from build123d import *

# Parameters (mm, degrees)
ESBO_O1_W                = 45
ESBO_O1_H                = 50
RESSALTO_EXTRUS_O1_DEPTH = 10
CORTE_EXTRUS_O1_DEPTH    = 7
CORTE_EXTRUS_O2_DEPTH    = 5.5
CHANFRO1_SIZE            = 5.5
ESBO_O4_R                = 1.65
RESSALTO_EXTRUS_O2_DEPTH = 3
CORTE_EXTRUS_O3_DEPTH    = 43.793106922


with BuildPart() as part:
    # Esboço1 → Ressalto-extrusão1 (new body)
    with BuildSketch(Plane.XY):
        Rectangle(ESBO_O1_W, ESBO_O1_H)
    extrude(amount=RESSALTO_EXTRUS_O1_DEPTH)

    # Esboço2 → Corte-extrusão1 (cut)
    with BuildSketch(Plane.XY.offset(10)):
        Polygon((-15, -5), (0, -12), (15, -5), (15, 25), (-15, 25), align=None)
    extrude(amount=-CORTE_EXTRUS_O1_DEPTH, mode=Mode.SUBTRACT)

    # Esboço3 → Corte-extrusão2 (cut)
    with BuildSketch(Plane.XY.offset(3)):
        Polygon((-15, -5), (-15, -12), (0, -19), (15, -12), (15, -5), align=None)
    extrude(amount=CORTE_EXTRUS_O2_DEPTH, mode=Mode.SUBTRACT)

    # Chanfro1
    chanfro1_edges = [part.edges().sort_by_distance(p)[0] for p in [
        (-7.5, -15.5, 8.5),
        (7.5, -15.5, 8.5),
    ]]
    chamfer(chanfro1_edges, length=CHANFRO1_SIZE - 0.0001)  # a hair under: the kernel refuses the full size

    # Esboço4 → Ressalto-extrusão2 (add)
    with BuildSketch(Plane(origin=(0, 0, 0), x_dir=(-1, 0, 0), z_dir=(0, 0, -1))):
        with BuildLine():
            Line((4.245283019, 32.641509434), (9, 25))
            Line((9, 25), (-9, 25))
            Line((-9, 25), (-4.245283019, 32.641509434))
            ThreePointArc((-4.245283019, 32.641509434), (0, 35), (4.245283019, 32.641509434))
        make_face()
        with Locations((0, 30)):
            Circle(ESBO_O4_R, mode=Mode.SUBTRACT)
    extrude(amount=-RESSALTO_EXTRUS_O2_DEPTH)

    # Esboço5 → Corte-extrusão3 (cut, through all)
    with BuildSketch(Plane.XY.offset(10)):
        Polygon((-22.5, -11.431767214), (0, -21.931767214), (22.5, -11.431767214), (22.5, -32.501990612), (-22.5, -32.501990612), align=None)
    extrude(amount=-CORTE_EXTRUS_O3_DEPTH, mode=Mode.SUBTRACT)


solid = part.part
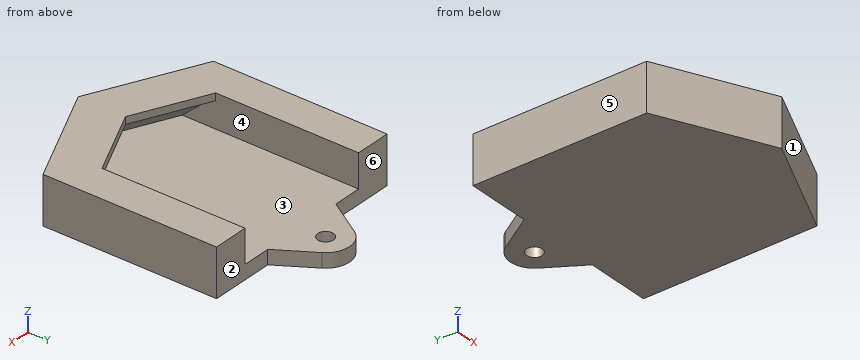
Here's how the part is built. I have some questions about the finished solid (model axes, mm). Face numbers are marked on the shaded views. A direction names the side the tool comes from. Give positions to 0.01 mm unless a question says otherwise; leave off trailing zeros. Loops run counter-clockwise (first coordinate to the right, second up) from the corner with the lowest first, then second, coordinate; pieces in that order, holes last. Notation, with made-up numbers: (29, 88.5) -> (75, 88.5) arc R35 cw to (75, 121.5) -> close; hole circle Ø6 at (0.25, -23.75). An arc over 180 degrees is marked (long way). Answer as a JSON object with one key per item and string values. Group by question number.
Item 1: Imagine slicing it at C-C on y = 30. Write out the boundary of the cut face in (x, z), then the cut area to 3 significant figures.
Item 2: Will these pins go through, and if not, where does the flat tip stop? pin 1 (6.5 mm diameter, centred on x = -1.5, y = -7.5, fed in from -Z); pin 2 (15 mm diameter, centred on x = 6.5, y = 17, fed in from +Z); pin 3 (4 mm diameter, centred on x = -2.5, z = 7.5, fed in from +Y); pin 4 (1.5 mm diameter, centred on x = 4, z = 5, fed in from -Y).
Item 3: Imagine slicing it at A-A on z = 1. Write out the boundary of the cut face in (x, y).
Item 4: On a 3-axis mill with a long thin cutter (end or side, diameter ignored), from which of +Z, -Z, +X, -X, +Y, -Y can I reach the whole of each face in a straight line? I mean the marked faces 4, 5 and 6. Say none if no direction works.
Item 5: Thinking about a two-plate mould opening in Y: for the marked faces 1, 2 and 3, which applies, pulls with the +Y half, pulls with the -Y half, needs draft (parallel to the pull), parting line crosses it, or undercut?
Item 6: I need wall thicknesses on L1, parallel to X at y = 17.5, z = 6.5; L2, parallel to Y at x = 0, z = 1.65; L3, parallel to Z at x = -2, y = 6.5. Which ranges of each line are inside material? Lowest first, please.
Answer list:
{
 "1": {"outline": "(-5.89, 0) -> (-1.65, 0) -> (-1.65, 3) -> (-5.89, 3) -> close; (1.65, 0) -> (5.89, 0) -> (5.89, 3) -> (1.65, 3) -> close", "area": "25.4 mm2"},
 "2": {"pin 1": "stops at z = 0", "pin 2": "stops at z = 3", "pin 3": "stops at y = -10.03", "pin 4": "stops at y = -20.42"},
 "3": {"outline": "(-22.5, -11.43) -> (0, -21.93) -> (22.5, -11.43) -> (22.5, 25) -> (9, 25) -> (4.25, 32.64) arc R5 ccw to (-4.25, 32.64) -> (-9, 25) -> (-22.5, 25) -> close; hole circle Ø3.3 at (0, 30)"},
 "4": {"face 4": "+Y", "face 5": "+Z, -Z, -X, +Y, -Y", "face 6": "+Z, -Z, -X, +Y"},
 "5": {"face 1": "pulls with the -Y half", "face 2": "pulls with the +Y half", "face 3": "needs draft"},
 "6": {"L1": "x = -22.5 to -15, 15 to 22.5", "L2": "y = -21.93 to 28.35, 31.65 to 35", "L3": "z = 0 to 3"}
}
